CAD build for the part. Positions are in the model's coordinates, mm. Face numbers are marked on the shaded views. Round coordinates to 2 decimals unless told otherwise and drop trailing zeros. Loops run counter-clockwise (first coordinate to the right, second up) from the corner with the lowest first, then second, coordinate; pieces in that order, holes last. Notation, with made-up numbers: (-17.5, 38) - (-1.5, 38) arc R21 cw to (-1.5, 68) - close; hole circle Ø7 at (36.25, -13). An arc over 180 degrees is marked (long way). Use one line per item in the form item = value.
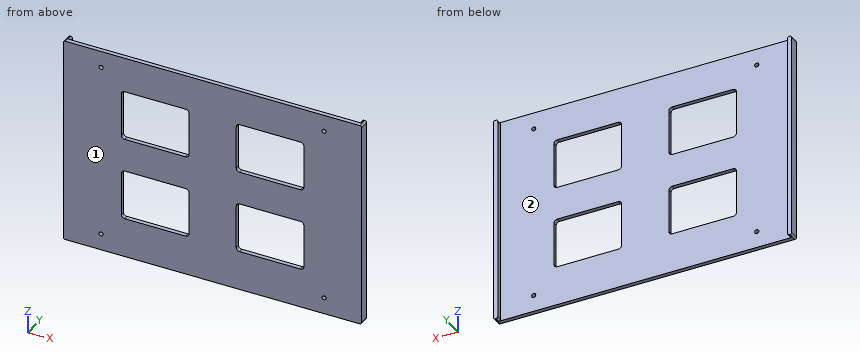
from build123d import *

# Parameters (mm, degrees)
SKETCH1_W                = 171.45
SKETCH1_H                = 125
SKETCH1_R                = 1.23
BOSS_EXTRUDE1_DEPTH      = 2.5
BOSS_EXTRUDE2_DEPTH      = 3
BOSS_EXTRUDE2_DEPTH_BACK = 2.5
SKETCH2_W                = 2.5
SKETCH2_H                = 125
CUT_EXTRUDE1_DEPTH       = 215.225587874
CUT_EXTRUDE1_DEPTH_BACK  = 215.225587874
SKETCH3_W                = 40
SKETCH3_H                = 30
FILLET1_R                = 2
FILLET2_R                = 1


with BuildPart() as part:
    # Sketch1 → Boss-Extrude1 (new body)
    with BuildSketch(Plane(origin=(0, 0, 0), x_dir=(1, 0, 0), z_dir=(0, 1, 0))):
        with Locations((85.725, -62.5)):
            Rectangle(SKETCH1_W, SKETCH1_H)
        with Locations(Location((19.725, -10, 0), (0, 0, 270))):
            Circle(SKETCH1_R, mode=Mode.SUBTRACT)
        with Locations(Location((151.725, -10, 0), (0, 0, 270))):
            Circle(SKETCH1_R, mode=Mode.SUBTRACT)
        with Locations(Location((19.725, -115, 0), (0, 0, 270))):
            Circle(SKETCH1_R, mode=Mode.SUBTRACT)
        with Locations(Location((151.725, -115, 0), (0, 0, 270))):
            Circle(SKETCH1_R, mode=Mode.SUBTRACT)
    extrude(amount=BOSS_EXTRUDE1_DEPTH)

    # Sketch2 → Boss-Extrude2 (add, two sides: drawn at the far end of the back side and taken through both)
    with BuildSketch(Plane(origin=(0, 2.5, 0), x_dir=(1, 0, 0), z_dir=(0, 1, 0)).offset(-BOSS_EXTRUDE2_DEPTH_BACK)):
        with Locations((-1.25, -62.5)):
            Rectangle(SKETCH2_W, SKETCH2_H)
        with Locations((172.7, -62.5)):
            Rectangle(SKETCH2_W, SKETCH2_H)
    extrude(amount=BOSS_EXTRUDE2_DEPTH + BOSS_EXTRUDE2_DEPTH_BACK)

    # Sketch3 → Cut-Extrude1 (cut, two sides: drawn at the far end of the back side and taken through both)
    with BuildSketch(Plane(origin=(0, 2.5, 0), x_dir=(1, 0, 0), z_dir=(0, 1, 0)).offset(-CUT_EXTRUDE1_DEPTH_BACK)):
        with Locations((51.725, -38.876953358)):
            Rectangle(SKETCH3_W, SKETCH3_H)
        with Locations((119.725, -38.876953358)):
            Rectangle(SKETCH3_W, SKETCH3_H)
        with Locations((51.725, -88.876953358)):
            Rectangle(SKETCH3_W, SKETCH3_H)
        with Locations((119.725, -88.876953358)):
            Rectangle(SKETCH3_W, SKETCH3_H)
    extrude(amount=CUT_EXTRUDE1_DEPTH + CUT_EXTRUDE1_DEPTH_BACK, mode=Mode.SUBTRACT)

    # Fillet1
    fillet1_edges = [part.edges().sort_by_distance(p)[0] for p in [
        (71.725, 1.25, 53.876953358),
        (139.725, 1.25, 23.876953358),
        (139.725, 1.25, 53.876953358),
        (99.725, 1.25, 53.876953358),
        (99.725, 1.25, 23.876953358),
        (31.725, 1.25, 103.876953358),
        (31.725, 1.25, 73.876953358),
        (71.725, 1.25, 73.876953358),
        (71.725, 1.25, 103.876953358),
        (99.725, 1.25, 103.876953358),
        (99.725, 1.25, 73.876953358),
        (139.725, 1.25, 73.876953358),
        (139.725, 1.25, 103.876953358),
        (31.725, 1.25, 53.876953358),
        (31.725, 1.25, 23.876953358),
        (71.725, 1.25, 23.876953358),
    ]]
    fillet(fillet1_edges, radius=FILLET1_R)

    # Fillet2
    fillet2_edges = [part.edges().sort_by_distance(p)[0] for p in [
        (0, 4, 0),
        (0, 4, 125),
        (-2.5, 2.75, 125),
        (-2.5, 2.75, 0),
        (171.45, 4, 125),
        (171.45, 4, 0),
        (173.95, 2.75, 0),
        (173.95, 2.75, 125),
    ]]
    fillet(fillet2_edges, radius=FILLET2_R)


solid = part.part
1) Flat gauge pins, fed straight in: pin 1 (3 mm diameter, centred on x = 19.725, z = 10, fed in from +Y); pin 2 (1.5 mm diameter, centred on x = 102, z = 35, fed in from +Y). Where does each tip first touch, or does it go through?
Report:
pin_1 = 2.5
pin_2 = through
2) Two-plate mould, pull along X, no slides. Class the marked faces 1 and 2: +X half, -X half, draft (parallel to the pull), parting line (faces both ways), or undercut.
Report:
face_1 = draft
face_2 = undercut
3) Slice it at D-D (x = 90.5). Write the cut outline in (y, z).
Report:
outline = (0, 0) - (2.5, 0) - (2.5, 125) - (0, 125) - close
4) Slice it at C-C (z = 21.5). Write the cut outline in (x, y), plus the area to 3 significant figures.
Report:
outline = (-2.5, 0) - (173.95, 0) - (173.95, 5.5) - (171.45, 5.5) - (171.45, 2.5) - (0, 2.5) - (0, 5.5) - (-2.5, 5.5) - close
area = 456 mm^2
5) Drill centre lines: probe 1 along X at (y, z) = (0.6, 115) (3 decimals); probe 2 along Z at (x, y) = (65, 0.65); probe 3 along X at (y, z) = (5.3, 108.5). Where is each one in solid material? Low to high.
Report:
probe_1 = -2.5 to 18.495, 20.955 to 150.495, 152.955 to 173.95
probe_2 = 0 to 23.88, 53.88 to 73.88, 103.88 to 125
probe_3 = -2.5 to 0, 171.45 to 173.95
6) Slice it at B-B (x = 43). Write the cut outline in (y, z), plus the area to 4 significant figures.
Report:
outline = (0, 0) - (2.5, 0) - (2.5, 23.88) - (0, 23.88) - close; (0, 53.88) - (2.5, 53.88) - (2.5, 73.88) - (0, 73.88) - close; (0, 103.88) - (2.5, 103.88) - (2.5, 125) - (0, 125) - close
area = 162.5 mm^2
7) Slice it at A-A (y = 3.5). Write the cut outline in (x, z).
Report:
outline = (-2.5, 1) arc R1 ccw to (-1.5, 0) - (-1, 0) arc R1 ccw to (0, 1) - (0, 124) arc R1 ccw to (-1, 125) - (-1.5, 125) arc R1 ccw to (-2.5, 124) - close; (171.45, 1) arc R1 ccw to (172.45, 0) - (172.95, 0) arc R1 ccw to (173.95, 1) - (173.95, 124) arc R1 ccw to (172.95, 125) - (172.45, 125) arc R1 ccw to (171.45, 124) - close
